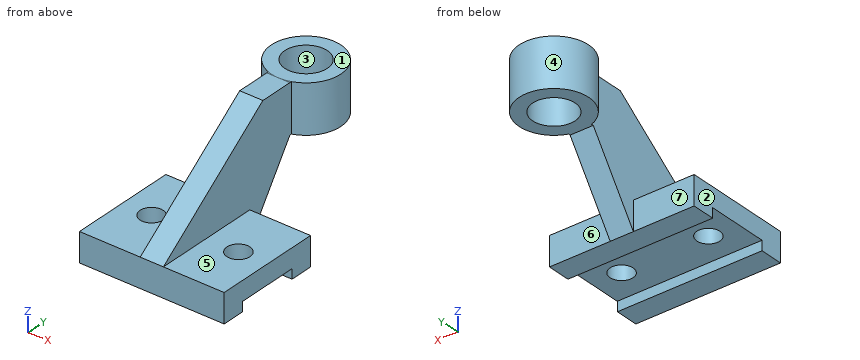
from build123d import *

# Parameters (mm, degrees)
F1_DEPTH = 37.5
F2_R     = 6
F3_DEPTH = 25
F5_DEPTH = 6
F7_R     = 18
F7_R_2   = 11
F8_DEPTH = 25


with BuildPart() as f1:
    # F0 (on Right) → F1 (new body, symmetric)
    with BuildSketch(Plane.YZ):
        Polygon((28, 0), (-28, 0), (-28, -15), (-16, -15), (-16, -10), (16, -10), (16, -15), (28, -15), align=None)
    extrude(amount=F1_DEPTH, both=True)

    # F2 (on face) → F3 (cut)
    with BuildSketch(Plane.XY):
        with Locations((-22.5, 0)):
            Circle(F2_R)
        with Locations((22.5, 0)):
            Circle(F2_R)
    extrude(amount=-F3_DEPTH, mode=Mode.SUBTRACT)

    # F4 (on Right) → F5 (join, symmetric)
    with BuildSketch(Plane.YZ):
        Polygon((54, 48), (36.491035, 48), (-28, 0), (28, 0), (28, -15), (54, 23), (59, 23), (59, 47.966335), align=None)
    extrude(amount=F5_DEPTH, both=True)

    # F7 (on offset) → F8 (join)
    with BuildSketch(Plane.XY.offset(48)):
        with Locations((0, 72)):
            Circle(F7_R)
        with Locations((0, 72)):
            Circle(F7_R_2, mode=Mode.SUBTRACT)
    extrude(amount=-F8_DEPTH)


solid = f1.part
Could you check a few things on this model? Use its own coordinates, in mm. Face numbers are marked on the shaded views. A direction names the side the tool comes from. Round coordinates to 2 decimals unless told otherwise and drop trailing zeros. Write each loop counter-clockwise with the first axis right and the second up, starting at its lowest first coordinate (ties: lowest second). Pieces come first, ordered by that corner, then holes. Notation, with made-up numbers: (4.5, 60) - (40.5, 60) arc R12 cw to (40.5, 64) - close; hole circle Ø6 at (66.5, 16.25). An arc over 180 degrees is marked (long way). Put each result on its own line as item: value. Start each with the question number.
(1) I want a section at C-C, the plane x = -31. Please give me the cut outline in (y, z).
(2) I want a section at D-D, the plane y = 0. Please give me the cut outline in (x, z).
(3) For the marked faces 5, 6 and 7, which set-ups out of +Z, -Z, +X, -X, +Y, -Y let a thin tool reach every point of the face, with its end or its side?
(4) Thinking about a two-plate mould opening in X: for the marked faces 1, 2, 3 and 4, which applies, released by +X, released by -X, zero draft, split by the parting line, or undercut?
(5) I need wall thicknesses on probe 1 along Y at (x, z) = (22.5, -3); probe 2 along Y at (x, z) = (-20.5, -10.5); probe 3 along X at (y, z) = (24, 24.5). Which ranges of each line are inside material? Lowest first, please.
(6) I want a section at B-B, the plane y = 72. Please give me the cut outline in (x, z), plus the area to 3 significant figures.
(7) Will these pins go through, and if not, where does the flat tip stop? pin 1 (12 mm diameter, centred on y = 35, z = -3.5, fed in from -X); pin 2 (18 mm diameter, centred on x = 4.5, y = 65, fed in from -Z); pin 3 (14 mm diameter, centred on x = 22.5, y = 0, fed in from +Z).
(8) I want a section at A-A, the plane x = 22.5. Please give me the cut outline in (y, z).
Here are the results:
1. outline: (-28, -15) - (-16, -15) - (-16, -10) - (16, -10) - (16, -15) - (28, -15) - (28, 0) - (-28, 0) - close
2. outline: (-37.5, -10) - (-28.5, -10) - (-28.5, 0) - (-37.5, 0) - close; (-16.5, -10) - (16.5, -10) - (16.5, 0) - (6, 0) - (6, 20.84) - (-6, 20.84) - (-6, 0) - (-16.5, 0) - close; (28.5, -10) - (37.5, -10) - (37.5, 0) - (28.5, 0) - close
3. face 5: +Z, +X, +Y, -Y
3. face 6: +Z, -Z, +X, +Y
3. face 7: +Z, -Z, -X, +Y
4. face 1: zero draft
4. face 2: released by -X
4. face 3: undercut
4. face 4: split by the parting line
5. probe 1: y = -28 to -6, 6 to 28
5. probe 2: y = -28 to -16, 16 to 28
5. probe 3: x = -6 to 6
6. outline: (-18, 23) - (-11, 23) - (-11, 48) - (-18, 48) - close; (11, 23) - (18, 23) - (18, 48) - (11, 48) - close
6. area: 350 mm^2
7. pin 1: stops at x = -6
7. pin 2: stops at z = 23
7. pin 3: stops at z = 0
8. outline: (-28, -15) - (-16, -15) - (-16, -10) - (-6, -10) - (-6, 0) - (-28, 0) - close; (6, -10) - (16, -10) - (16, -15) - (28, -15) - (28, 0) - (6, 0) - close
